```python
from build123d import *

# Parameters (mm, degrees)
F1_DEPTH = 19.05
F3_DEPTH = 25.4
F4_W     = 88.9
F4_H     = 19.05
F5_DEPTH = 19.05


with BuildPart() as f1:
    # F0 (on Front) → F1 (new body)
    with BuildSketch(Plane.XZ):
        with BuildLine():
            Line((754.452639, -127), (1219.750957, -127))
            Line((1219.750957, -127), (1218.132401, 0.307838))
            ThreePointArc((1218.132401, 0.307838), (971.957472, -30.969021), (754.452639, 88.496394))
            Line((754.452639, 88.496394), (754.452639, -127))
        make_face()
        with BuildLine():
            Line((152.950957, -127), (754.452639, -127))
            Line((754.452639, -127), (754.452639, 88.496394))
            ThreePointArc((754.452639, 88.496394), (389.486399, 159.988648), (152.950957, -127))
        make_face()
    extrude(amount=F1_DEPTH)

    # F2 (on face) → F3 (cut)
    with BuildSketch(Plane.XZ.offset(19.05)):
        Polygon((349.289218, -69.85), (250.3214, 41.61797), (186.588, -69.85), (250.3214, -69.85), (313.393829, -69.85), (314.054799, -69.85), align=None)
        Polygon((398.772179, 33.915376), (456.774034, 116.646986), (488.145278, 161.393719), (263.171888, 55.837033), (275.35156, 42.119006), (321.764452, -10.156076), (345.300821, -36.665212), (347.074358, -38.662755), (347.578352, -39.105525), (349.289218, -36.665212), align=None)
        Polygon((511.990437, 162.220746), (368.339218, -69.85), (655.641655, -69.85), align=None)
        Polygon((535.835596, 161.393719), (558.164751, 129.544273), (618.046186, 44.131702), (675.804029, -38.251859), (682.479221, -32.387854), (696.510871, -16.584994), (738.856518, 31.105928), (760.812477, 55.83338), align=None)
        Polygon((837.392874, -69.85), (773.662731, 41.614158), (674.691655, -69.85), align=None)
    extrude(amount=-F3_DEPTH, mode=Mode.SUBTRACT)

    # F4 (on face) → F5 (join)
    with BuildSketch(Plane.XZ.offset(19.05)):
        with Locations((705.400957, -136.525)):
            Rectangle(F4_W, F4_H)
        with Locations((273.600957, -136.525)):
            Rectangle(F4_W, F4_H)
        with Locations((489.500957, -136.525)):
            Rectangle(F4_W, F4_H)
    extrude(amount=-F5_DEPTH)


solid = f1.part
```
Model file for the job. Use its own axes, mm. A direction names the side the tool comes from. Coordinates: 2 decimals unless noted, no trailing zeros. Write each loop counter-clockwise with the first axis right and the second up, starting at its lowest first coordinate (ties: lowest second). Pieces come first, ordered by that corner, then holes. Notation, with made-up numbers: (33, 16.25) - (60, 16.25) arc R24 cw to (60, 55.25) - close; hole circle Ø8 at (5.5, -14.75). An arc over 180 degrees is marked (long way). One line per item, written item: value. Start each with the question number.
1. Mould opens along Z. For faces 5 (the cylindrical face through (975.43, -9.392, -31.614)), 6 (the flat face through (273, -10, -146.05)), 7 (the flat face through (805.974, -9.658, -14.898)) say: released by +Z, released by -Z, zero draft, split by the parting line, or undercut.
2. Tool access for faces 1 (the flat face through (229.151, -10, -137)), 2 (the flat face through (679, -19.05, -53)), 3 (the flat face through (597, -9, -127)), 4 (the flat face through (377.233, -9.658, 109.354)): list every direction of +Z, -Z, +X, -X, +Y, -Y with a clear straight run to the whole face (end or side of a thin tool).
3. Slice it at A-A (z = 69.5). Write the cut outline in (x, y), plus the area to 3 significant figures.
4. Flat gauge pins, fed straight in: pin 1 (5 mm diameter, centred on x = 780.5, y = -8.5, fed in from -Z); pin 2 (5.5 mm diameter, centred on x = 460, y = -7, fed in from +Z); pin 3 (5 mm diameter, centred on y = -9, z = 34, fed in from +X). Where does each tip first touch, or does it go through?
5. Slice it at B-B (x = 298). Write the cut outline in (y, z).
6. Slice it at C-C (y = -11.5). Count the separate pieces of the cut face and the enclosed holes in it, plus the area to 3 significant figures.
7. Slice it at D-D (z = 19). Write the cut outline in (x, y).
8. Probe line 1 (Z direction, x = 592, y = -15.5); line 2 (Z direction, x = 601, y = -12); line 3 (X direction, y = -9.5, z = 71). List the from-to ranges inside material, lowest first. Write a range as from..to.
Answers below:
1. face 5: released by +Z
1. face 6: released by -Z
1. face 7: undercut
2. face 1: -Z, -X, +Y, -Y
2. face 2: +Z, -Z, +X, -X, -Y
2. face 3: -Z, +Y, -Y
2. face 4: +Y, -Y
3. outline: (249.88, -19.05) - (292.29, -19.05) - (292.29, 0) - (249.88, 0) - close; (423.72, -19.05) - (454.6, -19.05) - (454.6, 0) - (423.72, 0) - close; (569.38, -19.05) - (600.26, -19.05) - (600.26, 0) - (569.38, 0) - close; (731.69, -19.05) - (773.54, -19.05) - (773.54, 0) - (731.69, 0) - close
3. area: 2,780 mm^2
4. pin 1: stops at z = -127
4. pin 2: stops at z = 177.92
4. pin 3: stops at x = 821.16
5. outline: (-19.05, -146.05) - (0, -146.05) - (0, -69.85) - (-19.05, -69.85) - close; (-19.05, -12.08) - (0, -12.08) - (0, 16.61) - (-19.05, 16.61) - close; (-19.05, 72.18) - (0, 72.18) - (0, 111.54) - (-19.05, 111.54) - close
6. separate pieces: 1
6. enclosed holes: 5
6. area: 130,000 mm^2
7. outline: (209.42, -19.05) - (237.39, -19.05) - (237.39, 0) - (209.42, 0) - close; (270.4, -19.05) - (295.88, -19.05) - (295.88, 0) - (270.4, 0) - close; (388.32, -19.05) - (423.34, -19.05) - (423.34, 0) - (388.32, 0) - close; (600.64, -19.05) - (635.67, -19.05) - (635.67, 0) - (600.64, 0) - close; (728.11, -19.05) - (753.58, -19.05) - (753.58, 0) - (728.11, 0) - close; (786.59, -19.05) - (840.72, -19.05) - (840.72, 0) - (786.59, 0) - close
8. line 1: z = -127..-69.85, 32.96..81.28, 135.04..172.35
8. line 2: z = -127..-69.85, 18.42..68.45, 130.82..170.2
8. line 3: x = 251.33..295.49, 424.77..455.53, 568.46..599.21, 728.49..771.94
